from build123d import *

# Parameters (mm, degrees)
CROQUIS1_R              = 24
CROQUIS1_R_2            = 1.5
SALIENTE_EXTRUIR1_DEPTH = 13
REDONDEO1_R             = 2
REDONDEO2_R             = 2


with BuildPart() as part:
    # Croquis1 → Saliente-Extruir1 (new body)
    with BuildSketch(Plane.XY):
        with Locations(Location((-49.242561536, 14.193667069, 0), (0, 0, 180))):
            Circle(CROQUIS1_R)
        with Locations(Location((-49.242561536, 14.193667069, 0), (0, 0, 180))):
            Circle(CROQUIS1_R_2, mode=Mode.SUBTRACT)
    extrude(amount=SALIENTE_EXTRUIR1_DEPTH)

    # Redondeo1
    redondeo1_edges = [part.edges().sort_by_distance(p)[0] for p in [
        (-25.242561536, 14.193667069, 13),
    ]]
    fillet(redondeo1_edges, radius=REDONDEO1_R)

    # Redondeo2
    redondeo2_edges = [part.edges().sort_by_distance(p)[0] for p in [
        (-25.242561536, 14.193667069, 0),
    ]]
    fillet(redondeo2_edges, radius=REDONDEO2_R)


solid = part.part
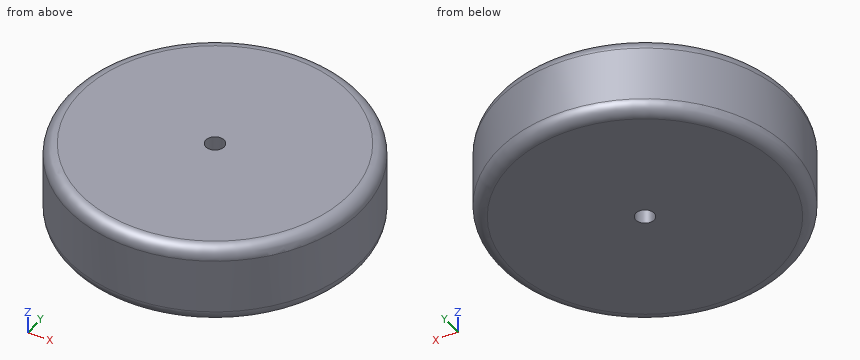
Input: part model. Units: mm. Frame: model coordinates. Coordinates: 2 decimals unless noted, no trailing zeros. Order: outer loops, then holes, each group sorted by start corner. A loop starts at its lowest first (then second) coordinate and runs counter-clockwise, first axis right, second up. Notation, with made-up numbers: M 48,15 L 56,15 A16 ccw 56,41 Z; hole C 75,-1.5 d1. An arc over 180 degrees is marked long. Write item = value, one per line. Start each with the question number.
(1) Section A-A on z = 8.25. Output: boundary loops of the cut face in (x, y), and give its area (3 significant figures).
(2) First-contact query: P1, Ø5, axis at y = 25.5, z = 8, coming from the +X side; P2, Ø5, axis at x = -46.5, z = 6, coming from the -Y side; P3, Ø6, axis at x = -55.5, z = 8, coming from the -Y side. Flat tips, straight axial feed; report the tip coordinate or a pass-through.
(3) Line query: line 1 along Y through (x, z) = (-49.5, 12); line 2 along X through (y, z) = (15, 11.25); line 3 along Y through (x, z) = (-48, 5). Output: solid intervals per line, ascending. Write a range as [from, to].
Result set:
q1.outline = C -49.24,14.19 d48; hole C -49.24,14.19 d3
q1.area = 1,800 mm²
q2.P1 = -26.92
q2.P2 = -9.81
q2.P3 = -9.58
q3.line_1 = [-9.54, 12.72], [15.67, 37.92]
q3.line_2 = [-73.21, -50.51], [-47.98, -25.27]
q3.line_3 = [-9.77, 13.35], [15.03, 38.16]
